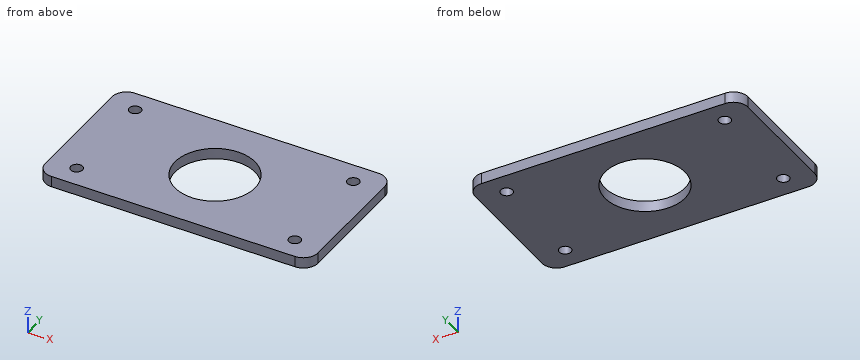
```python
from build123d import *

# Parameters (mm, degrees)
SKETCH2_W               = 150
SKETCH2_H               = 80
BOSS_EXTRUDE1_DEPTH     = 3
CUT_EXTRUDE1_DEPTH      = 86.211501571
CUT_EXTRUDE1_DEPTH_BACK = 86.211501571
SKETCH3_R               = 3.25
SKETCH3_R_2             = 22
FILLET2_R               = 8


with BuildPart() as part:
    # Sketch2 → Boss-Extrude1 (new, symmetric)
    with BuildSketch(Plane.XY):
        Rectangle(SKETCH2_W, SKETCH2_H)
    extrude(amount=BOSS_EXTRUDE1_DEPTH, both=True)

    # Sketch3 → Cut-Extrude1 (cut, two sides: drawn at the far end of the back side and taken through both)
    with BuildSketch(Plane.XY.offset(3).offset(-CUT_EXTRUDE1_DEPTH_BACK)):
        with Locations((-60, 28)):
            Circle(SKETCH3_R)
        with Locations((-60, -28)):
            Circle(SKETCH3_R)
        with Locations((60, -28)):
            Circle(SKETCH3_R)
        with Locations((60, 28)):
            Circle(SKETCH3_R)
        Circle(SKETCH3_R_2)
    extrude(amount=CUT_EXTRUDE1_DEPTH + CUT_EXTRUDE1_DEPTH_BACK, mode=Mode.SUBTRACT)

    # Fillet2
    fillet2_edges = [part.edges().sort_by_distance(p)[0] for p in [
        (75, -40, 0),
        (-75, -40, 0),
        (-75, 40, 0),
        (75, 40, 0),
    ]]
    fillet(fillet2_edges, radius=FILLET2_R)


solid = part.part
```
The model under review builds one solid part; all positions refer to its coordinate system, in mm. Coordinates: 2 decimals unless noted, no trailing zeros. Write each loop counter-clockwise with the first axis right and the second up, starting at its lowest first coordinate (ties: lowest second). Pieces come first, ordered by that corner, then holes. Notation, with made-up numbers: (-13, -23) - (9, -23) arc R33 ccw to (9, 6) - close; hole circle Ø10 at (29, 61.5). An arc over 180 degrees is marked (long way). Answer in a Markdown table with one row per item. Add a question column.
Q1. Consider section D-D on x = -60. Give the boundary of the cut face in (y, z).
Q2. Consider section B-B on y = 28. Give the boundary of the cut face in (x, z), then the cut area to 3 significant figures.
Q3. To check wall thickness, follow line 1 along Y through (x, z) = (-60, -0.95); line 2 along X through (y, z) = (28, 0.45); line 3 along X through (y, z) = (-1, -2.7). State the ranges of each line that lie inside material, in increasing order. Write a range as from..to.
Q4. Clearance check with flat-ended pins moving along their axes: pin 1 (4 mm diameter, centred on x = 60, y = -28, fed in from +Z); pin 2 (8.5 mm diameter, centred on x = -60, y = 28, fed in from -Z). State where each tip first meets the part, or that it passes through.
Q5. Consider section A-A on x = 0. Give the boundary of the cut face in (y, z).
Q6. Consider section C-C on z = 0.75. Give the boundary of the cut face in (x, y).
Answers below:
| question | item | result |
|---|---|---|
| 1 | outline | (-40, -3) - (-31.25, -3) - (-31.25, 3) - (-40, 3) - close; (-24.75, -3) - (24.75, -3) - (24.75, 3) - (-24.75, 3) - close; (31.25, -3) - (40, -3) - (40, 3) - (31.25, 3) - close |
| 2 | outline | (-75, -3) - (-63.25, -3) - (-63.25, 3) - (-75, 3) - close; (-56.75, -3) - (56.75, -3) - (56.75, 3) - (-56.75, 3) - close; (63.25, -3) - (75, -3) - (75, 3) - (63.25, 3) - close |
| 2 | area | 822 mm² |
| 3 | line 1 | -40..-31.25, -24.75..24.75, 31.25..40 |
| 3 | line 2 | -75..-63.25, -56.75..56.75, 63.25..75 |
| 3 | line 3 | -75..-21.98, 21.98..75 |
| 4 | pin 1 | through |
| 4 | pin 2 | z = -3 |
| 5 | outline | (-40, -3) - (-22, -3) - (-22, 3) - (-40, 3) - close; (22, -3) - (40, -3) - (40, 3) - (22, 3) - close |
| 6 | outline | (-75, -32) arc R8 ccw to (-67, -40) - (67, -40) arc R8 ccw to (75, -32) - (75, 32) arc R8 ccw to (67, 40) - (-67, 40) arc R8 ccw to (-75, 32) - close; hole circle Ø6.5 at (-60, -28); hole circle Ø6.5 at (-60, 28); hole circle Ø44 at (0, 0); hole circle Ø6.5 at (60, -28); hole circle Ø6.5 at (60, 28) |
